from build123d import *

# Parameters (mm, degrees)
ESQUISSE1_W              = 48
ESQUISSE1_H              = 31
BOSS_EXTRU_1_DEPTH       = 3
ENL_V_MAT_EXTRU_2_REACH  = 59.219
ESQUISSE3_W              = 10
ESQUISSE3_H              = 3
ENL_V_MAT_EXTRU_3_REACH  = 59.219
ESQUISSE4_W              = 5.5
ESQUISSE4_H              = 3
ENL_V_START              = -3
ESQUISSE5_W              = 3.5
ESQUISSE5_H              = 11
ENL_V_MAT_EXTRU_4_DEPTH  = 3
ENL_V_MAT_EXTRU_7_REACH  = 59.219
ESQUISSE8_W              = 5
ESQUISSE8_H              = 3
ENL_V_MAT_EXTRU_8_REACH  = 59.219
ESQUISSE9_W              = 5
ESQUISSE9_H              = 3
ENL_V_MAT_EXTRU_14_REACH = 59.219
ESQUISSE18_W             = 4
ESQUISSE18_H             = 3
ENL_V_MAT_EXTRU_19_REACH = 59.219
ESQUISSE23_W             = 4
ESQUISSE23_H             = 3
ENL_V_MAT_EXTRU_20_REACH = 59.219
ENL_V_MAT_EXTRU_21_REACH = 59.219
ESQUISSE25_W             = 19
ESQUISSE25_H             = 3
ENL_V_MAT_EXTRU_22_REACH = 59.219
ESQUISSE26_W             = 19
ESQUISSE26_H             = 3
ENL_V_MAT_EXTRU_23_REACH = 59.219
ESQUISSE27_R             = 8
ENL_V_MAT_EXTRU_24_REACH = 59.219
ESQUISSE28_R             = 8
ESQUISSE29_R             = 2
BOSS_EXTRU_5_DEPTH       = 4
ESQUISSE30_R             = 2
BOSS_EXTRU_6_DEPTH       = 4
ENL_V_MAT_EXTRU_25_REACH = 59.567
ESQUISSE31_R             = 0.75
ENL_V_MAT_EXTRU_26_REACH = 59.567
ESQUISSE32_R             = 0.75
BOSS_EXTRU_7_DEPTH       = 4
BOSS_EXTRU_8_DEPTH       = 4
ENL_V_MAT_EXTRU_27_REACH = 59.567
ENL_V_MAT_EXTRU_29_REACH = 59.567
CHANFREIN4_SIZE          = 5
CHANFREIN5_SIZE          = 4


with BuildPart() as part:
    # Esquisse1 → Boss.-Extru.1 (new body)
    with BuildSketch(Plane.XY):
        with Locations((24, 15.5)):
            Rectangle(ESQUISSE1_W, ESQUISSE1_H)
    extrude(amount=BOSS_EXTRU_1_DEPTH)

    # Esquisse3 → Enlèv. mat.-Extru.2 (cut, up to next)
    with BuildSketch(Plane.XY.offset(3), mode=Mode.PRIVATE) as enl_v_mat_extru_2_sk1:
        with Locations((24, 1.5)):
            Rectangle(ESQUISSE3_W, ESQUISSE3_H)
    enl_v_mat_extru_2_tool1 = extrude(enl_v_mat_extru_2_sk1.sketch, amount=-ENL_V_MAT_EXTRU_2_REACH, mode=Mode.PRIVATE) & part.part
    add(enl_v_mat_extru_2_tool1.solids().sort_by_distance((24, 1.5, 3))[0], mode=Mode.SUBTRACT)

    # Esquisse4 → Enlèv. mat.-Extru.3 (cut, up to next)
    with BuildSketch(Plane.XY.offset(3), mode=Mode.PRIVATE) as enl_v_mat_extru_3_sk1:
        with Locations((24, 7.5)):
            Rectangle(ESQUISSE4_W, ESQUISSE4_H)
    enl_v_mat_extru_3_tool1 = extrude(enl_v_mat_extru_3_sk1.sketch, amount=-ENL_V_MAT_EXTRU_3_REACH, mode=Mode.PRIVATE) & part.part
    add(enl_v_mat_extru_3_tool1.solids().sort_by_distance((24, 7.5, 3))[0], mode=Mode.SUBTRACT)

    # Esquisse5 → Enlèv. mat.-Extru.4 (cut)
    with BuildSketch(Plane.XY.offset(3).offset(ENL_V_START)):
        with Locations((24, 5.5)):
            Rectangle(ESQUISSE5_W, ESQUISSE5_H)
    extrude(amount=ENL_V_MAT_EXTRU_4_DEPTH, mode=Mode.SUBTRACT)

    # Esquisse8 → Enlèv. mat.-Extru.7 (cut, up to next)
    with BuildSketch(Plane.XY.offset(3), mode=Mode.PRIVATE) as enl_v_mat_extru_7_sk1:
        with Locations((2.5, 1.5)):
            Rectangle(ESQUISSE8_W, ESQUISSE8_H)
    enl_v_mat_extru_7_tool1 = extrude(enl_v_mat_extru_7_sk1.sketch, amount=-ENL_V_MAT_EXTRU_7_REACH, mode=Mode.PRIVATE) & part.part
    add(enl_v_mat_extru_7_tool1.solids().sort_by_distance((2.5, 1.5, 3))[0], mode=Mode.SUBTRACT)

    # Esquisse9 → Enlèv. mat.-Extru.8 (cut, up to next)
    with BuildSketch(Plane.XY.offset(3), mode=Mode.PRIVATE) as enl_v_mat_extru_8_sk1:
        with Locations((45.5, 1.5)):
            Rectangle(ESQUISSE9_W, ESQUISSE9_H)
    enl_v_mat_extru_8_tool1 = extrude(enl_v_mat_extru_8_sk1.sketch, amount=-ENL_V_MAT_EXTRU_8_REACH, mode=Mode.PRIVATE) & part.part
    add(enl_v_mat_extru_8_tool1.solids().sort_by_distance((45.5, 1.5, 3))[0], mode=Mode.SUBTRACT)

    # Esquisse18 → Enlèv. mat.-Extru.14 (cut, up to next)
    with BuildSketch(Plane.XY.offset(3), mode=Mode.PRIVATE) as enl_v_mat_extru_14_sk1:
        with Locations((41, 1.5)):
            Rectangle(ESQUISSE18_W, ESQUISSE18_H)
    enl_v_mat_extru_14_tool1 = extrude(enl_v_mat_extru_14_sk1.sketch, amount=-ENL_V_MAT_EXTRU_14_REACH, mode=Mode.PRIVATE) & part.part
    add(enl_v_mat_extru_14_tool1.solids().sort_by_distance((41, 1.5, 3))[0], mode=Mode.SUBTRACT)

    # Esquisse23 → Enlèv. mat.-Extru.19 (cut, up to next)
    with BuildSketch(Plane.XY.offset(3), mode=Mode.PRIVATE) as enl_v_mat_extru_19_sk1:
        with Locations((7, 1.5)):
            Rectangle(ESQUISSE23_W, ESQUISSE23_H)
    enl_v_mat_extru_19_tool1 = extrude(enl_v_mat_extru_19_sk1.sketch, amount=-ENL_V_MAT_EXTRU_19_REACH, mode=Mode.PRIVATE) & part.part
    add(enl_v_mat_extru_19_tool1.solids().sort_by_distance((7, 1.5, 3))[0], mode=Mode.SUBTRACT)

    # Esquisse24 → Enlèv. mat.-Extru.20 (cut, up to next)
    with BuildSketch(Plane.XY.offset(3), mode=Mode.PRIVATE) as enl_v_mat_extru_20_sk1:
        Polygon((20, 22), (24, 26), (28, 22), align=None)
    enl_v_mat_extru_20_tool1 = extrude(enl_v_mat_extru_20_sk1.sketch, amount=-ENL_V_MAT_EXTRU_20_REACH, mode=Mode.PRIVATE) & part.part
    add(enl_v_mat_extru_20_tool1.solids().sort_by_distance((24, 23.333333, 3))[0], mode=Mode.SUBTRACT)

    # Esquisse25 → Enlèv. mat.-Extru.21 (cut, up to next)
    with BuildSketch(Plane.XY.offset(3), mode=Mode.PRIVATE) as enl_v_mat_extru_21_sk1:
        with Locations((38.5, 29.5)):
            Rectangle(ESQUISSE25_W, ESQUISSE25_H)
    enl_v_mat_extru_21_tool1 = extrude(enl_v_mat_extru_21_sk1.sketch, amount=-ENL_V_MAT_EXTRU_21_REACH, mode=Mode.PRIVATE) & part.part
    add(enl_v_mat_extru_21_tool1.solids().sort_by_distance((38.5, 29.5, 3))[0], mode=Mode.SUBTRACT)

    # Esquisse26 → Enlèv. mat.-Extru.22 (cut, up to next)
    with BuildSketch(Plane.XY.offset(3), mode=Mode.PRIVATE) as enl_v_mat_extru_22_sk1:
        with Locations((9.5, 29.5)):
            Rectangle(ESQUISSE26_W, ESQUISSE26_H)
    enl_v_mat_extru_22_tool1 = extrude(enl_v_mat_extru_22_sk1.sketch, amount=-ENL_V_MAT_EXTRU_22_REACH, mode=Mode.PRIVATE) & part.part
    add(enl_v_mat_extru_22_tool1.solids().sort_by_distance((9.5, 29.5, 3))[0], mode=Mode.SUBTRACT)

    # Esquisse27 → Enlèv. mat.-Extru.23 (cut, up to next)
    with BuildSketch(Plane.XY.offset(3), mode=Mode.PRIVATE) as enl_v_mat_extru_23_sk1:
        with Locations((38, 15)):
            Circle(ESQUISSE27_R)
    enl_v_mat_extru_23_tool1 = extrude(enl_v_mat_extru_23_sk1.sketch, amount=-ENL_V_MAT_EXTRU_23_REACH, mode=Mode.PRIVATE) & part.part
    add(enl_v_mat_extru_23_tool1.solids().sort_by_distance((38, 15, 3))[0], mode=Mode.SUBTRACT)

    # Esquisse28 → Enlèv. mat.-Extru.24 (cut, up to next)
    with BuildSketch(Plane.XY.offset(3), mode=Mode.PRIVATE) as enl_v_mat_extru_24_sk1:
        with Locations((10, 15)):
            Circle(ESQUISSE28_R)
    enl_v_mat_extru_24_tool1 = extrude(enl_v_mat_extru_24_sk1.sketch, amount=-ENL_V_MAT_EXTRU_24_REACH, mode=Mode.PRIVATE) & part.part
    add(enl_v_mat_extru_24_tool1.solids().sort_by_distance((10, 15, 3))[0], mode=Mode.SUBTRACT)

    # Esquisse29 → Boss.-Extru.5 (add)
    with BuildSketch(Plane.XY.offset(3)):
        with Locations(Location((4, 24, 0), (0, 0, 180))):
            Circle(ESQUISSE29_R)
    extrude(amount=BOSS_EXTRU_5_DEPTH)

    # Esquisse30 → Boss.-Extru.6 (add)
    with BuildSketch(Plane.XY.offset(3)):
        with Locations(Location((44, 24, 0), (0, 0, 180))):
            Circle(ESQUISSE30_R)
    extrude(amount=BOSS_EXTRU_6_DEPTH)

    # Esquisse31 → Enlèv. mat.-Extru.25 (cut, up to next)
    with BuildSketch(Plane.XY.offset(7), mode=Mode.PRIVATE) as enl_v_mat_extru_25_sk1:
        with Locations((4, 24)):
            Circle(ESQUISSE31_R)
    enl_v_mat_extru_25_tool1 = extrude(enl_v_mat_extru_25_sk1.sketch, amount=-ENL_V_MAT_EXTRU_25_REACH, mode=Mode.PRIVATE) & part.part
    add(enl_v_mat_extru_25_tool1.solids().sort_by_distance((4, 24, 7))[0], mode=Mode.SUBTRACT)

    # Esquisse32 → Enlèv. mat.-Extru.26 (cut, up to next)
    with BuildSketch(Plane.XY.offset(7), mode=Mode.PRIVATE) as enl_v_mat_extru_26_sk1:
        with Locations((44, 24)):
            Circle(ESQUISSE32_R)
    enl_v_mat_extru_26_tool1 = extrude(enl_v_mat_extru_26_sk1.sketch, amount=-ENL_V_MAT_EXTRU_26_REACH, mode=Mode.PRIVATE) & part.part
    add(enl_v_mat_extru_26_tool1.solids().sort_by_distance((44, 24, 7))[0], mode=Mode.SUBTRACT)

    # Esquisse33 → Boss.-Extru.7 (add)
    with BuildSketch(Plane.XY.offset(3)):
        with BuildLine():
            Line((3, 9), (4, 9))
            ThreePointArc((4, 9), (6, 7), (4, 5))
            Line((4, 5), (3, 5))
            ThreePointArc((3, 5), (1, 7), (3, 9))
        make_face()
    extrude(amount=BOSS_EXTRU_7_DEPTH)

    # Esquisse34 → Boss.-Extru.8 (add)
    with BuildSketch(Plane.XY.offset(3)):
        with BuildLine():
            Line((44, 9), (45, 9))
            ThreePointArc((45, 9), (47, 7), (45, 5))
            Line((45, 5), (44, 5))
            ThreePointArc((44, 5), (42, 7), (44, 9))
        make_face()
    extrude(amount=BOSS_EXTRU_8_DEPTH)

    # Esquisse35 → Enlèv. mat.-Extru.27 (cut, up to next)
    with BuildSketch(Plane.XY.offset(7), mode=Mode.PRIVATE) as enl_v_mat_extru_27_sk1:
        with BuildLine():
            Line((3, 7.75), (4, 7.75))
            ThreePointArc((4, 7.75), (4.75, 7), (4, 6.25))
            Line((4, 6.25), (3, 6.25))
            ThreePointArc((3, 6.25), (2.25, 7), (3, 7.75))
        make_face()
    enl_v_mat_extru_27_tool1 = extrude(enl_v_mat_extru_27_sk1.sketch, amount=-ENL_V_MAT_EXTRU_27_REACH, mode=Mode.PRIVATE) & part.part
    add(enl_v_mat_extru_27_tool1.solids().sort_by_distance((3.5, 7, 7))[0], mode=Mode.SUBTRACT)

    # Esquisse37 → Enlèv. mat.-Extru.29 (cut, up to next)
    with BuildSketch(Plane.XY.offset(7), mode=Mode.PRIVATE) as enl_v_mat_extru_29_sk1:
        with BuildLine():
            Line((44, 7.75), (45, 7.75))
            ThreePointArc((45, 7.75), (45.75, 7), (45, 6.25))
            Line((45, 6.25), (44, 6.25))
            ThreePointArc((44, 6.25), (43.25, 7), (44, 7.75))
        make_face()
    enl_v_mat_extru_29_tool1 = extrude(enl_v_mat_extru_29_sk1.sketch, amount=-ENL_V_MAT_EXTRU_29_REACH, mode=Mode.PRIVATE) & part.part
    add(enl_v_mat_extru_29_tool1.solids().sort_by_distance((44.5, 7, 7))[0], mode=Mode.SUBTRACT)

    # Chanfrein4
    chanfrein4_edges = [part.edges().sort_by_distance(p)[0] for p in [
        (48, 28, 1.5),
        (0, 28, 1.5),
    ]]
    chamfer(chanfrein4_edges, length=CHANFREIN4_SIZE)

    # Chanfrein5
    chanfrein5_edges = [part.edges().sort_by_distance(p)[0] for p in [
        (0, 3, 1.5),
        (48, 3, 1.5),
    ]]
    chamfer(chanfrein5_edges, length=CHANFREIN5_SIZE)


solid = part.part
Input: part model. Units: mm. Frame: model coordinates. A direction names the side the tool comes from. Give positions to 0.01 mm unless a question says otherwise; leave off trailing zeros. Order: outer loops, then holes, each group sorted by start corner. A loop starts at its lowest first (then second) coordinate and runs counter-clockwise, first axis right, second up.
Q1. Section C-C on x = 23. Output: boundary loops of the cut face in (y, z), and give its area (3 significant figures).
Checked values:
outline: (11, 0) - (22, 0) - (22, 3) - (11, 3) - close; (25, 0) - (31, 0) - (31, 3) - (25, 3) - close
area: 51.0 mm2
Q2. Set-up query: faces 1 (the cylindrical face through (4.75, 7.02, 3.55)), 2 (the flat face through (44.5, 9, 5)), 3 (the flat face through (25.75, 10, 1)). Return all of +Z, -Z, +X, -X, +Y, -Y with unobstructed straight access to the full face (end or side cutting, diameter ignored); none if empty.
Checked values:
face 1: +Z, -Z
face 2: +Z, +X, -X
face 3: +Z, -Z, -Y
Q3. Section B-B on y = 24. Output: boundary loops of the cut face in (x, z), and give its area (3 significant figures).
Checked values:
outline: (1, 0) - (3.25, 0) - (3.25, 7) - (2, 7) - (2, 3) - (1, 3) - close; (4.75, 0) - (22, 0) - (22, 3) - (6, 3) - (6, 7) - (4.75, 7) - close; (26, 0) - (43.25, 0) - (43.25, 7) - (42, 7) - (42, 3) - (26, 3) - close; (44.75, 0) - (47, 0) - (47, 3) - (46, 3) - (46, 7) - (44.75, 7) - close
area: 137 mm2
Q4. Ray query, probe 1 along X at (y, z) = (15, 2.4); probe 2 along Y at (x, z) = (10, 1.05); probe 3 along X at (y, z) = (13.5, 1.5). Return the intervals inside material, ascending.
Checked values:
probe 1: x = 0 to 2, 18 to 30, 46 to 48
probe 2: y = 0 to 7, 23 to 28
probe 3: x = 0 to 2.14, 17.86 to 30.14, 45.86 to 48
Q5. Section D-D on y = 15. Output: boundary loops of the cut face in (x, z).
Checked values:
outline: (0, 0) - (2, 0) - (2, 3) - (0, 3) - close; (18, 0) - (30, 0) - (30, 3) - (18, 3) - close; (46, 0) - (48, 0) - (48, 3) - (46, 3) - close
Q6. Draft query along Y for faces 4 (the flat face through (0, 15, 1)), 5 (the flat face through (14, 0, 1)), 6 (the flat face through (21.25, 7, 2)). Return one class per face: +Y half, -Y half, draft (parallel to the pull), parting line (faces both ways), or undercut.
Checked values:
face 4: draft
face 5: -Y half
face 6: undercut
Q7. Section A-A on z = 6. Output: boundary loops of the cut face in (x, y), and give its area (3 significant figures).
Checked values:
outline: circle Ø4 at (4, 24); (3, 5) - (4, 5) arc R2 ccw to (4, 9) - (3, 9) arc R2 ccw to start; circle Ø4 at (44, 24); (44, 5) - (45, 5) arc R2 ccw to (45, 9) - (44, 9) arc R2 ccw to start; hole (3, 6.25) - (4, 6.25) arc R0.75 ccw to (4, 7.75) - (3, 7.75) arc R0.75 ccw to start; hole circle Ø1.5 at (4, 24); hole circle Ø1.5 at (44, 24); hole (44, 6.25) - (45, 6.25) arc R0.75 ccw to (45, 7.75) - (44, 7.75) arc R0.75 ccw to start
area: 48.2 mm2
Q8. Contact query for flat-ended pins moving along their axis: pin 1 Ø0.9 at (x, z) = (20.5, 2) entering from -Y; pin 2 Ø3.5 at (y, z) = (2, 1.5) entering from -X; pin 3 Ø12 at (x, y) = (28, 5) entering from +Z; pin 4 Ø1.5 at (y, z) = (14, 5.5) entering from -X. Output: stop coordinate, or through.
Checked values:
pin 1: stops at y = 3
pin 2: stops at x = 3.25
pin 3: stops at z = 3
pin 4: passes through
